from build123d import *

# Parameters (mm, degrees)
EXTRUDE_1_DEPTH      = 2.9
SKETCH_2_R           = 3.4
EXTRUDE_2_DEPTH      = 1.1
SKETCH_3_R           = 2
CUT_EXTRUDE_1_DEPTH  = 7.555404895
SKETCH_2_2_OUTSIDE_W = 13.226
SKETCH_2_2_OUTSIDE_H = 14.278
SKETCH_2_2_OUTSIDE_R = 3.4
CUT_EXTRUDE_2_DEPTH  = 1.1
CUT_EXTRUDE_2_DRAFT  = -45
SKETCH_4_OUTSIDE_W   = 13.226
SKETCH_4_OUTSIDE_H   = 14.278
SKETCH_4_OUTSIDE_R   = 3.4
CUT_EXTRUDE_3_DEPTH  = 1.1
CUT_EXTRUDE_3_DRAFT  = -45
FILLET_1_R           = 0.3


with BuildPart() as part:
    # Sketch 1 → Extrude 1 (new body)
    with BuildSketch(Plane.XY):
        Polygon((0, 3.92598183), (-3.4, 1.962990915), (-3.4, -1.962990915), (0, -3.92598183), (3.4, -1.962990915), (3.4, 1.962990915), align=None)
    extrude(amount=EXTRUDE_1_DEPTH)

    # Sketch 2 → Extrude 2 (add)
    with BuildSketch(Plane.XY.offset(2.9)):
        Circle(SKETCH_2_R)
    extrude(amount=EXTRUDE_2_DEPTH)

    # Sketch 3 → Cut-Extrude 1 (cut, through all)
    with BuildSketch(Plane.XY.offset(4)):
        Circle(SKETCH_3_R)
    extrude(amount=-CUT_EXTRUDE_1_DEPTH, mode=Mode.SUBTRACT)


with BuildPart() as cut_extrude_2_tool:
    # Sketch 2_2 outside → Cut-Extrude 2 (with draft: the straight prism first)
    with BuildSketch(Plane.XY.offset(2.9)):
        Rectangle(SKETCH_2_2_OUTSIDE_W, SKETCH_2_2_OUTSIDE_H)
        Circle(SKETCH_2_2_OUTSIDE_R, mode=Mode.SUBTRACT)
    extrude(amount=-CUT_EXTRUDE_2_DEPTH)
    # Cut-Extrude 2: the draft: its side faces are tilted about the plane it starts from
    cut_extrude_2_sides = [cut_extrude_2_tool.faces().sort_by_distance(p)[0] for p in [
        (0, -7.139, 2.35),
        (6.613, 0, 2.35),
        (0, 7.139, 2.35),
        (-6.613, 0, 2.35),
        (-3.4, 0, 2.35),
    ]]
    draft(cut_extrude_2_sides, Plane.XY.offset(2.9), CUT_EXTRUDE_2_DRAFT)


with BuildPart() as part_1:
    add(part.part)

    # Cut-Extrude 2: cut by cut_extrude_2_tool
    add(cut_extrude_2_tool.part, mode=Mode.SUBTRACT)


with BuildPart() as cut_extrude_3_tool:
    # Sketch 4 outside → Cut-Extrude 3 (with draft: the straight prism first)
    with BuildSketch(Plane(origin=(0, 0, 0), x_dir=(-1, 0, 0), z_dir=(0, 0, -1))):
        Rectangle(SKETCH_4_OUTSIDE_W, SKETCH_4_OUTSIDE_H)
        with Locations(Location((0, 0, 0), (0, 0, 180))):
            Circle(SKETCH_4_OUTSIDE_R, mode=Mode.SUBTRACT)
    extrude(amount=-CUT_EXTRUDE_3_DEPTH)
    # Cut-Extrude 3: the draft: its side faces are tilted about the plane it starts from
    cut_extrude_3_sides = [cut_extrude_3_tool.faces().sort_by_distance(p)[0] for p in [
        (0, -7.139, 0.55),
        (-6.613, 0, 0.55),
        (0, 7.139, 0.55),
        (6.613, 0, 0.55),
        (-3.4, 0, 0.55),
    ]]
    draft(cut_extrude_3_sides, Plane(origin=(0, 0, 0), x_dir=(-1, 0, 0), z_dir=(0, 0, -1)), CUT_EXTRUDE_3_DRAFT)


with BuildPart() as part_2:
    add(part_1.part)

    # Cut-Extrude 3: cut by cut_extrude_3_tool
    add(cut_extrude_3_tool.part, mode=Mode.SUBTRACT)

    # Fillet 1
    fillet_1_edges = [part_2.edges().sort_by_distance(p)[0] for p in [
        (-3.4, 0, 4),
    ]]
    fillet(fillet_1_edges, radius=FILLET_1_R)


solid = part_2.part
Design review of the part built by this model. Coordinates are the model's own, in mm. A direction names the side the tool comes from. Give positions to 0.01 mm unless a question says otherwise; leave off trailing zeros. Loops run counter-clockwise (first coordinate to the right, second up) from the corner with the lowest first, then second, coordinate; pieces in that order, holes last. Notation, with made-up numbers: (-34.5, 50) - (-4.5, 50) arc R30 ccw to (-4.5, 78) - close; hole circle Ø2 at (30.25, -14). An arc over 180 degrees is marked (long way). Use CSV: the item, a comma, the result in double quotes. Start each with the question number.
1. Machinability: for faces 1 (the conical face through (3.06, -1.76, 0.13)), 2 (the cylindrical face through (-0.74, -3.32, 3.29)), which of the approach directions +Z, -Z, +X, -X, +Y, -Y give a long, thin tool a straight path to every point of the face, cutting with its end or side? Answer none if there is none.
2. Add section A-A (z = 1.6). State the section outline as (x, y) points.
3. Draft analysis for pull direction Y (two halves, no side actions). For faces 3 (the cylindrical face through (0, -2, 2)), 4 (the conical face through (0.01, 3.53, 2.77)), 5 (the conical face through (-3.049, -1.77, 0.125)), 6 (the flat face through (2, -1, 4)), state which applies: released by +Y, released by -Y, zero draft, split by the parting line, or undercut.
4. Add section B-B (z = 2.5). State the section outline as (x, y) points, plus the area to 3 significant figures.
5. Wall thickness on L1, parallel to X at y = -1.25, z = 0.5; L2, parallel to X at y = 0.5, z = 0.75; L3, parallel to Y at x = -0.25, z = 3.2: over which ranges is each line inside the solid? List them lowest first.
6. Add section C-C (z = 3.3). State the section outline as (x, y) points, plus the area to 3 significant figures.
7. Insertion check: P1, Ø2, axis at x = -2.5, z = 1.5, coming from the +Y side; P2, Ø1, axis at x = -0.5, z = 3.5, coming from the -Y side. Each pin has a flat end and moves straight along its axis. Give the tip position at first contact, or say it passes through.
Results found:
1,face 1,"-Z, +X, -Y"
1,face 2,"+Z"
2,outline,"(-3.4, -1.96) - (0, -3.93) - (3.4, -1.96) - (3.4, 1.96) - (0, 3.93) - (-3.4, 1.96) - close; hole circle Ø4 at (0, 0)"
3,face 3,"undercut"
3,face 4,"released by +Y"
3,face 5,"released by -Y"
3,face 6,"zero draft"
4,outline,"(-3.4, -1.7) arc R3.8 ccw to (-3.17, -2.1) - (-0.23, -3.79) arc R3.8 ccw to (0.23, -3.79) - (3.17, -2.1) arc R3.8 ccw to (3.4, -1.7) - (3.4, 1.7) arc R3.8 ccw to (3.17, 2.1) - (0.23, 3.79) arc R3.8 ccw to (-0.23, 3.79) - (-3.17, 2.1) arc R3.8 ccw to (-3.4, 1.7) - close; hole circle Ø4 at (0, 0)"
4,area,"27.3 mm²"
5,L1,"x = -3.4 to -1.56, 1.56 to 3.4"
5,L2,"x = -3.4 to -1.94, 1.94 to 3.4"
5,L3,"y = -3.39 to -1.98, 1.98 to 3.39"
6,outline,"circle Ø6.8 at (0, 0); hole circle Ø4 at (0, 0)"
6,area,"23.8 mm²"
7,P1,"stops at y = 3.06"
7,P2,"stops at y = -3.4"
